from build123d import *

# Parameters (mm, degrees)
SKETCH1_R           = 8.5
BOSS_EXTRUDE1_DEPTH = 5
SKETCH2_R           = 7.5
BOSS_EXTRUDE2_DEPTH = 10
SKETCH3_R           = 6.75
CUT_EXTRUDE1_DEPTH  = 5
BOSS_EXTRUDE5_DEPTH = 5
SKETCH5_R           = 6.270829758
SKETCH5_R_2         = 2.95954522
CUT_EXTRUDE2_DEPTH  = 1


with BuildPart() as part:
    # Sketch1 → Boss-Extrude1 (new body)
    with BuildSketch(Plane.XY):
        Circle(SKETCH1_R)
    extrude(amount=BOSS_EXTRUDE1_DEPTH)

    # Sketch2 → Boss-Extrude2 (add)
    with BuildSketch(Plane.XY.offset(5)):
        Circle(SKETCH2_R)
    extrude(amount=BOSS_EXTRUDE2_DEPTH)

    # Sketch3 → Cut-Extrude1 (cut)
    with BuildSketch(Plane.XY.offset(15)):
        Circle(SKETCH3_R)
    extrude(amount=-CUT_EXTRUDE1_DEPTH, mode=Mode.SUBTRACT)

    # Sketch4 → Boss-Extrude5 (add)
    with BuildSketch(Plane.XY.offset(15)):
        Polygon((-6.45, 0), (-6.877641054, 0.75), (-6.877641054, -0.75), align=None)
        Polygon((-6.067099227, 3.324868934), (-6.641124376, 1.939049636), (-5.959022985, 2.468308139), align=None)
        Polygon((-4.332896542, 5.393556714), (-5.393556714, 4.332896542), (-4.560838739, 4.560838739), align=None)
        Polygon((-1.939049636, 6.641124376), (-3.324868934, 6.067099227), (-2.468308139, 5.959022985), align=None)
        Polygon((0.75, 6.877641054), (-0.75, 6.877641054), (0, 6.45), align=None)
        Polygon((3.324868934, 6.067099227), (1.939049636, 6.641124376), (2.468308139, 5.959022985), align=None)
        Polygon((5.393556714, 4.332896542), (4.332896542, 5.393556714), (4.560838739, 4.560838739), align=None)
        Polygon((6.641124376, 1.939049636), (6.067099227, 3.324868934), (5.959022985, 2.468308139), align=None)
        Polygon((6.877641054, -0.75), (6.877641054, 0.75), (6.45, 0), align=None)
        Polygon((6.067099227, -3.324868934), (6.641124376, -1.939049636), (5.959022985, -2.468308139), align=None)
        Polygon((4.332896542, -5.393556714), (5.393556714, -4.332896542), (4.560838739, -4.560838739), align=None)
        Polygon((1.939049636, -6.641124376), (3.324868934, -6.067099227), (2.468308139, -5.959022985), align=None)
        Polygon((-0.75, -6.877641054), (0.75, -6.877641054), (0, -6.45), align=None)
        Polygon((-3.324868934, -6.067099227), (-1.939049636, -6.641124376), (-2.468308139, -5.959022985), align=None)
        Polygon((-5.393556714, -4.332896542), (-4.332896542, -5.393556714), (-4.560838739, -4.560838739), align=None)
        Polygon((-6.641124376, -1.939049636), (-6.067099227, -3.324868934), (-5.959022985, -2.468308139), align=None)
    extrude(amount=-BOSS_EXTRUDE5_DEPTH)

    # Sketch5 → Cut-Extrude2 (cut)
    with BuildSketch(Plane(origin=(0, 0, 0), x_dir=(-1, 0, 0), z_dir=(0, 0, -1))):
        Circle(SKETCH5_R)
        Circle(SKETCH5_R_2, mode=Mode.SUBTRACT)
    extrude(amount=-CUT_EXTRUDE2_DEPTH, mode=Mode.SUBTRACT)


solid = part.part
Check sheet for the modelled part. Datum: model origin and axes. Units: mm. A direction names the side the tool comes from. Round coordinates to 2 decimals unless told otherwise and drop trailing zeros. Loops run counter-clockwise (first coordinate to the right, second up) from the corner with the lowest first, then second, coordinate; pieces in that order, holes last. Notation, with made-up numbers: M -29,25.5 L 30,25.5 A30 cw 30,48.5 Z; hole C 71,38.5 d11. An arc over 180 degrees is marked long. One line per question, with ' | ' between items. Start each with the question number.
Item 1: Release check for a two-part mould opening along Y. For faces 4 (the face through (-3.74, 5.62, 12.54)), 5 (the face through (0, -8, 5)), 6 (the face through (4.57, 7.167, 2.465)) record: released by +Y, released by -Y, zero draft, split by the parting line, or undercut.
Item 2: Section check A-A (x = 3.75). Record the boundary of the cut face in (y, z).
Item 3: Gauge pin test, flat ends, axial feed: pin 1 Ø5 at (y, z) = (1, 6) entering from +X; pin 2 Ø6 at (y, z) = (0.5, 11.5) entering from -X; pin 3 Ø2 at (y, z) = (4, 9) entering from +X. Record the tip position at first contact, or that the pin passes through.
Item 4: Scan lines: probe 1 along Y at (x, z) = (0, 0.3); probe 2 along Z at (x, y) = (0.5, 4.5); probe 3 along X at (y, z) = (3.25, 10.25). Record each from-to range of solid material in increasing order.
Item 5: Section check B-B (z = 2.75). Record the boundary of the cut face in (x, y).
Item 6: Set-up check for faces 1 (the face through (0, 0, 0)), 2 (the face through (-1.31, 6.62, 12.54)), 3 (the face through (0.816, 6.217, 0.493)): record each of +Z, -Z, +X, -X, +Y, -Y from which the full face is reachable in a straight line by a thin tool's end or side.
Item 7: Section check D-D (x = -1.25). Record the boundary of the cut face in (y, z), and give its area (3 significant figures).
Item 8: Section check C-C (y = -1). Record the boundary of the cut face in (x, z), and give its area (3 significant figures).
Worked out:
1) face 4: undercut | face 5: zero draft | face 6: split by the parting line
2) outline: M -7.63,0 L -5.03,0 L -5.03,1 L 5.03,1 L 5.03,0 L 7.63,0 L 7.63,5 L 6.5,5 L 6.5,15 L 5.61,15 L 5.61,10 L -5.61,10 L -5.61,15 L -6.5,15 L -6.5,5 L -7.63,5 Z
3) pin 1: x = 8.5 | pin 2: x = -7.5 | pin 3: x = 6.87
4) probe 1: -8.5 to -6.27, -2.96 to 2.96, 6.27 to 8.5 | probe 2: 1 to 10 | probe 3: -6.76 to -5.92, 5.92 to 6.76
5) outline: C 0,0 d17
6) face 1: -Z, +X, -X, +Y, -Y | face 2: +Z | face 3: -Z
7) outline: M -8.41,0 L -6.14,0 L -6.14,1 L -2.68,1 L -2.68,0 L 2.68,0 L 2.68,1 L 6.14,1 L 6.14,0 L 8.41,0 L 8.41,5 L 7.4,5 L 7.4,15 L 6.63,15 L 6.63,10 L -6.63,10 L -6.63,15 L -7.4,15 L -7.4,5 L -8.41,5 Z | area: 159 mm^2
8) outline: M -8.44,0 L -6.19,0 L -6.19,1 L -2.79,1 L -2.79,0 L 2.79,0 L 2.79,1 L 6.19,1 L 6.19,0 L 8.44,0 L 8.44,5 L 7.43,5 L 7.43,15 L 6.68,15 L 6.68,10 L -6.68,10 L -6.68,15 L -7.43,15 L -7.43,5 L -8.44,5 Z | area: 160 mm^2
